from build123d import *

# Parameters (mm, degrees)
F0_W      = 16
F0_H      = 40
F1_DEPTH  = 16
F2_R      = 2.6
F3_DEPTH  = 5
F4_R      = 2.1
F5_DEPTH  = 5
F6_R      = 2.1
F7_DEPTH  = 5
F8_R      = 2.1
F9_DEPTH  = 5
F10_R     = 2.1
F11_DEPTH = 5
F12_R     = 1.25
F13_DEPTH = 1
F14_R     = 1.25
F15_DEPTH = 1
F16_R     = 1.25
F17_DEPTH = 1
F18_R     = 1.25
F19_DEPTH = 1
F21_DEPTH = 1
F22_R     = 0.9999
F23_DEPTH = 0.5


# Not quite as in the source:
# - a fillet or chamfer is up to 0.001 mm smaller than in the source, because OpenCascade refuses the exact size


with BuildPart() as f1:
    # F0 (on Front) → F1 (new body)
    with BuildSketch(Plane.XZ):
        Rectangle(F0_W, F0_H)
    extrude(amount=F1_DEPTH)

    # F2 (on face) → F3 (cut)
    with BuildSketch(Plane.XY.offset(20)):
        with Locations((0, -8)):
            Circle(F2_R)
    extrude(amount=-F3_DEPTH, mode=Mode.SUBTRACT)

    # F4 (on face) → F5 (cut)
    with BuildSketch(Plane.YZ.offset(8)):
        with Locations((-8, 10)):
            Circle(F4_R)
    extrude(amount=-F5_DEPTH, mode=Mode.SUBTRACT)

    # F6 (on face) → F7 (cut)
    with BuildSketch(Plane(origin=(-8, 0, 0), x_dir=(0, -1, 0), z_dir=(-1, 0, 0))):
        with Locations((8, 10)):
            Circle(F6_R)
    extrude(amount=-F7_DEPTH, mode=Mode.SUBTRACT)

    # F8 (on face) → F9 (cut)
    with BuildSketch(Plane(origin=(0, 0, -20), x_dir=(1, 0, 0), z_dir=(0, 0, -1))):
        with Locations((4, 8)):
            Circle(F8_R)
    extrude(amount=-F9_DEPTH, mode=Mode.SUBTRACT)

    # F10 (on face) → F11 (cut)
    with BuildSketch(Plane(origin=(0, 0, -20), x_dir=(1, 0, 0), z_dir=(0, 0, -1))):
        with Locations((-4, 8)):
            Circle(F10_R)
    extrude(amount=-F11_DEPTH, mode=Mode.SUBTRACT)

    # F12 (on face) → F13 (join)
    with BuildSketch(Plane.XZ.offset(16)):
        with Locations((0, 7)):
            Circle(F12_R)
    extrude(amount=F13_DEPTH)

    # F14 (on face) → F15 (join)
    with BuildSketch(Plane.XZ.offset(16)):
        with Locations((0, 2)):
            Circle(F14_R)
    extrude(amount=F15_DEPTH)

    # F16 (on face) → F17 (join)
    with BuildSketch(Plane.XZ.offset(16)):
        with Locations((0, -3)):
            Circle(F16_R)
    extrude(amount=F17_DEPTH)

    # F18 (on face) → F19 (join)
    with BuildSketch(Plane.XZ.offset(16)):
        with Locations((0, -8)):
            Circle(F18_R)
    extrude(amount=F19_DEPTH)

    # F20 (on face) → F21 (join)
    with BuildSketch(Plane.XZ.offset(16)):
        with BuildLine():
            add(Edge.make_bspline(
                [(0.75, 20), (3.3594071533, 20.0532824127), (5.9301231166, 20.3851114773), (8, 21)],
                knots=[8.72055047, 8.72055047, 8.72055047, 8.72055047, 16, 16, 16, 16], degree=3))
            Line((0.75, 20), (7.9315101276, 20))
            add(Edge.make_bspline(
                [(8, 21), (7.936682093, 20.7032053334), (7.9331222274, 20.3617292136), (7.9315101276, 20)],
                knots=[0, 0, 0, 0, 0.1427572475, 0.1427572475, 0.1427572475, 0.1427572475], degree=3))
        make_face()
        with BuildLine():
            add(Edge.make_bspline(
                [(-8, 21), (-5.9479143878, 20.3884393869), (-3.3741827757, 20.0535723375), (-0.75, 20)],
                knots=[0, 0, 0, 0, 7.3266434187, 7.3266434187, 7.3266434187, 7.3266434187], degree=3))
            add(Edge.make_bspline(
                [(-8, 21), (-7.9392027192, 20.7034220667), (-7.9347343847, 20.3618566303), (-7.9314905291, 20)],
                knots=[0, 0, 0, 0, 0.1427309242, 0.1427309242, 0.1427309242, 0.1427309242], degree=3))
            Line((-7.9314905291, 20), (-0.75, 20))
        make_face()
        with BuildLine():
            Line((7.9315101276, 20), (0.75, 20))
            add(Edge.make_bspline(
                [(1.5735535475, 17.5164310059), (1.3638279631, 18.3834931797), (1.1151249806, 19.2296253371), (0.75, 20)],
                knots=[4.0589797926, 4.0589797926, 4.0589797926, 4.0589797926, 6.690552617, 6.690552617, 6.690552617, 6.690552617], degree=3))
            add(Edge.make_bspline(
                [(2.55, 13.5561273817), (2.1277926475, 14.7918965335), (1.8970376255, 16.1790605143), (1.5735535475, 17.5164310059)],
                knots=[0, 0, 0, 0, 4.0589797926, 4.0589797926, 4.0589797926, 4.0589797926], degree=3))
            add(Edge.make_bspline(
                [(7.9315101276, 20), (7.9285658859, 19.3393596044), (7.9402465057, 16.9450971177), (4.2150295862, 15.4292771095), (2.55, 13.5561273817)],
                knots=[0.1427572475, 0.1427572475, 0.1427572475, 0.1427572475, 0.4034804652, 1, 1, 1, 1], degree=3))
        make_face()
        with BuildLine():
            add(Edge.make_bspline(
                [(-1.5894267657, 17.4658260078), (-1.3661758267, 18.3343166755), (-1.104863981, 19.193579629), (-0.75, 20)],
                knots=[4.0525124649, 4.0525124649, 4.0525124649, 4.0525124649, 6.690552617, 6.690552617, 6.690552617, 6.690552617], degree=3))
            Line((-0.75, 20), (-7.9314905291, 20))
            add(Edge.make_bspline(
                [(-7.9314905291, 20), (-7.9255644562, 19.3389382799), (-7.9195168056, 16.9429139448), (-4.3261046571, 15.4424536286), (-2.55, 13.5561273817)],
                knots=[0.1427309242, 0.1427309242, 0.1427309242, 0.1427309242, 0.4034804652, 1, 1, 1, 1], degree=3))
            add(Edge.make_bspline(
                [(-2.55, 13.5561273817), (-2.185517021, 14.7757286924), (-1.9323810655, 16.1316653987), (-1.5894267657, 17.4658260078)],
                knots=[0, 0, 0, 0, 4.0525124649, 4.0525124649, 4.0525124649, 4.0525124649], degree=3))
        make_face()
    extrude(amount=F21_DEPTH)

    # F22 (radius 1 in the source; OpenCascade refuses exactly that, so slightly less here)
    f22_edges = [f1.edges().sort_by_distance(p)[0] for p in [
        (4.408175, -17, 20.266958),
        (-4.589536, -17, 20.290754),
    ]]
    fillet(f22_edges, radius=F22_R)

    # F20 (on face) → F23 (join)
    with BuildSketch(Plane.XZ.offset(16)):
        with BuildLine():
            Line((0.75, 20), (-0.75, 20))
            add(Edge.make_bspline(
                [(-0.75, 20), (-0.2507445203, 19.9898077667), (0.2503370769, 19.9897972051), (0.75, 20)],
                knots=[7.3266434187, 7.3266434187, 7.3266434187, 7.3266434187, 8.72055047, 8.72055047, 8.72055047, 8.72055047], degree=3))
        make_face()
        with BuildLine():
            add(Edge.make_bspline(
                [(-0.75, 20), (-0.2507445203, 19.9898077667), (0.2503370769, 19.9897972051), (0.75, 20)],
                knots=[7.3266434187, 7.3266434187, 7.3266434187, 7.3266434187, 8.72055047, 8.72055047, 8.72055047, 8.72055047], degree=3))
            add(Edge.make_bspline(
                [(-1.5894267657, 17.4658260078), (-1.3661758267, 18.3343166755), (-1.104863981, 19.193579629), (-0.75, 20)],
                knots=[4.0525124649, 4.0525124649, 4.0525124649, 4.0525124649, 6.690552617, 6.690552617, 6.690552617, 6.690552617], degree=3))
            add(Edge.make_bspline(
                [(-1.5894267657, 17.4658260078), (-0.646941675, 17.3500761834), (0.6084956384, 17.4665004575), (1.5735535475, 17.5164310059)],
                knots=[0, 0, 0, 0, 3.1633851058, 3.1633851058, 3.1633851058, 3.1633851058], degree=3))
            add(Edge.make_bspline(
                [(1.5735535475, 17.5164310059), (1.3638279631, 18.3834931797), (1.1151249806, 19.2296253371), (0.75, 20)],
                knots=[4.0589797926, 4.0589797926, 4.0589797926, 4.0589797926, 6.690552617, 6.690552617, 6.690552617, 6.690552617], degree=3))
        make_face()
    extrude(amount=F23_DEPTH)


solid = f1.part
Could you check a few things on this model? Use its own coordinates, in mm. A direction names the side the tool comes from. Coordinates: 2 decimals unless noted, no trailing zeros. Order: outer loops, then holes, each group sorted by start corner. A loop starts at its lowest first (then second) coordinate and runs counter-clockwise, first axis right, second up.
Q1. Thinking about a two-plate mould opening in Y: for faces 4 (the flat face through (4, -8, -15)), 5 (the flat face through (0, 0, 0)), 6 (the flat face through (0, -17, 2)), which applies, released by +Y, released by -Y, zero draft, split by the parting line, or undercut?
Q2. Suppose I cut it at A-A on z = -3. Please give me the cut outline in (x, y).
Q3. Suppose I cut it at C-C on z = 10. Please give me the cut outline in (x, y), and give its area (3 significant figures).
Q4. Suppose I cut it at B-B on y = -8. Please give me the cut outline in (x, z).
Q5. Will these pins go through, and if not, where does the flat tip stop? pin 1 (3.5 mm diameter, centred on x = 4, y = -8, fed in from -Z); pin 2 (0.8 mm diameter, centred on x = -3.5, z = 20.5, fed in from +Y); pin 3 (4 mm diameter, centred on x = 4.5, z = 2.5, fed in from -Y).
Q6. Suppose I cut it at D-D on y = -11. Please give me the cut outline in (x, z).
Q7. Which directions (+Z, -Z, +X, -X, +Y, -Y) give clear straight access to the entire face, cutting with the end or side of a thin tool? Please do faces 1 (the flat face through (3, -8, 10)), 2 (the flat face through (-6, -16, 20.3)), 3 (the cylindrical face through (-0.56, -10.54, 17.54)).
Q8. Please list where these lines run through material, in increasing order: L1, parallel to Z at x = -5.95, y = -8; L2, parallel to Z at x = -3.5, y = -3.25; L3, parallel to Y at x = 7, z = 13.5.
Answer:
1. face 4: undercut
1. face 5: released by +Y
1. face 6: released by -Y
2. outline: (-8, -16) - (-1.25, -16) - (-1.25, -17) - (1.25, -17) - (1.25, -16) - (8, -16) - (8, 0) - (-8, 0) - close
3. outline: (-8, -16) - (8, -16) - (8, -10.1) - (3, -10.1) - (3, -5.9) - (8, -5.9) - (8, 0) - (-8, 0) - (-8, -5.9) - (-3, -5.9) - (-3, -10.1) - (-8, -10.1) - close
3. area: 214 mm2
4. outline: (-8, -20) - (-6.1, -20) - (-6.1, -15) - (-1.9, -15) - (-1.9, -20) - (1.9, -20) - (1.9, -15) - (6.1, -15) - (6.1, -20) - (8, -20) - (8, 7.9) - (3, 7.9) - (3, 12.1) - (8, 12.1) - (8, 20) - (2.6, 20) - (2.6, 15) - (-2.6, 15) - (-2.6, 20) - (-8, 20) - (-8, 12.1) - (-3, 12.1) - (-3, 7.9) - (-8, 7.9) - close
5. pin 1: stops at z = -15
5. pin 2: stops at y = -16
5. pin 3: stops at y = -16
6. outline: (-8, -20) - (8, -20) - (8, 20) - (-8, 20) - close
7. face 1: +X
7. face 2: +Z, +X, -X, +Y
7. face 3: +Z
8. L1: z = -15 to 7.9, 12.1 to 20
8. L2: z = -20 to 20
8. L3: y = -16 to 0
